Could you check a few things on this drawing? It's one solid part, dimensions in mm from its lowest x, y, z. Round coordinates to 2 decimals unless told otherwise and drop trailing zeros. Loops run counter-clockwise (first coordinate to the right, second up) from the corner with the lowest first, then second, coordinate; pieces in that order, holes last.
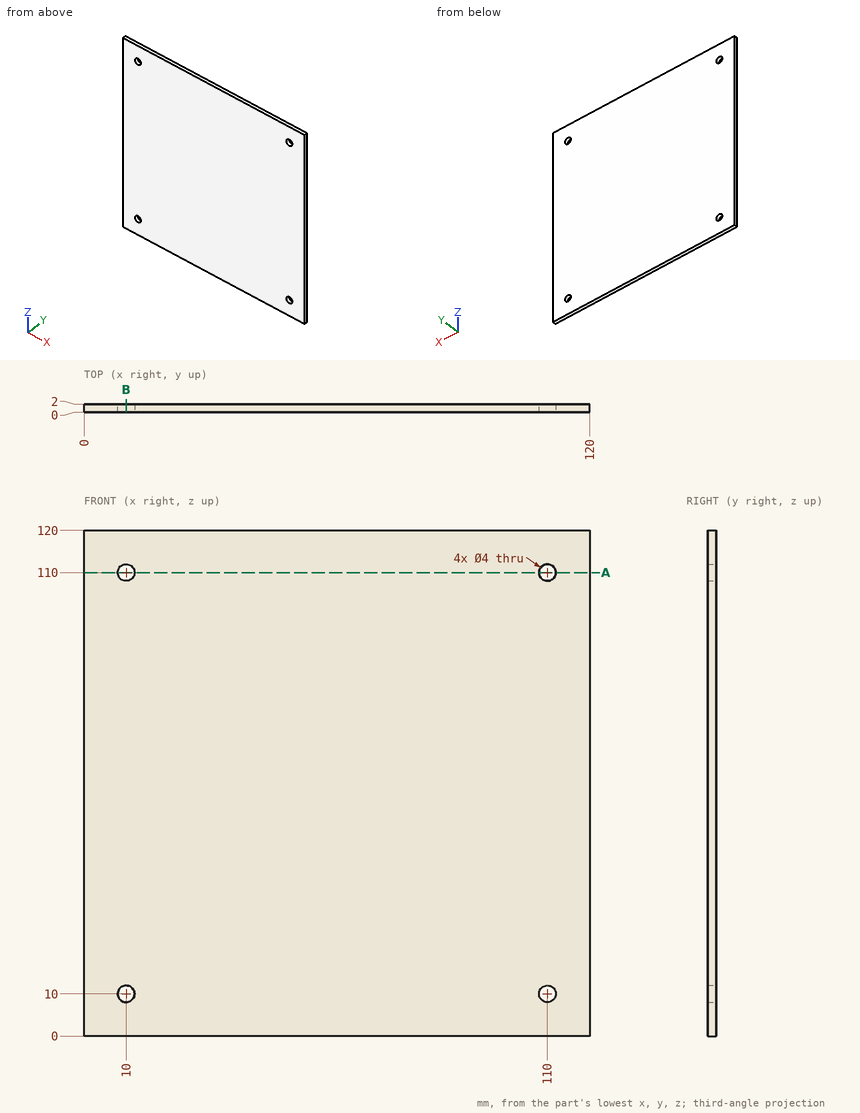
(1) Suppose I cut it at B-B (x = 10). Write out the boundary of the cut face in (y, z), then the cut area to 3 significant figures.
(2) If I drill on line 1 (X direction, y = 1.15, z = 10); line 2 (X direction, y = 0.2, z = 111.5), over which ranges is the centre line in solid material (lowest first)?
(3) Suppose I cut it at A-A (z = 110). Write out the boundary of the cut face in (x, y), then the cut area to 3 significant figures.
Check result:
1. outline: (0, 0) - (2, 0) - (2, 8) - (0, 8) - close; (0, 12) - (2, 12) - (2, 108) - (0, 108) - close; (0, 112) - (2, 112) - (2, 120) - (0, 120) - close
1. area: 224 mm2
2. line 1: x = 0 to 8, 12 to 108, 112 to 120
2. line 2: x = 0 to 8.68, 11.32 to 108.68, 111.32 to 120
3. outline: (0, 0) - (8, 0) - (8, 2) - (0, 2) - close; (12, 0) - (108, 0) - (108, 2) - (12, 2) - close; (112, 0) - (120, 0) - (120, 2) - (112, 2) - close
3. area: 224 mm2
